```python
from build123d import *

# Parameters (mm, degrees)
SKETCH1_R                         = 30.48
BOSS_EXTRUDE1_DEPTH               = 25.4
F_1_4_28_TAPPED_HOLE1_D           = 5.4102
SKETCH7_R                         = 11.43
CUT_EXTRUDE2_DEPTH                = 12.7
F_1_4_CLEARANCE_HOLE1_D           = 6.5278
F_1_4_NPT_TAPPED_HOLE1_AT_2_COUNT = 2
F_1_4_NPT_TAPPED_HOLE1_AT_2_PITCH = 40.7035
CUT_EXTRUDE3_DEPTH                = 12.7
GASKET_SLOT_DEPTH                 = 1.016


with BuildPart() as part:
    # Sketch1 → Boss-Extrude1 (new body)
    with BuildSketch(Plane(origin=(0, 0, 0), x_dir=(1, 0, 0), z_dir=(0, 1, 0))):
        with Locations(Location((0, 0, 0), (0, 0, 270))):
            Circle(SKETCH1_R)
    extrude(amount=BOSS_EXTRUDE1_DEPTH)

    # 1/4-28 Tapped Hole1 (through all)
    with Locations(Plane(origin=(0, 25.4, 0), x_dir=(1, 0, 0), z_dir=(0, 1, 0))):
        with Locations((0, 0)):
            Hole(F_1_4_28_TAPPED_HOLE1_D / 2)

    # Sketch7 → Cut-Extrude2 (cut)
    with BuildSketch(Plane.XZ):
        with Locations(Location((0, 0, 0), (0, 0, 270))):
            Circle(SKETCH7_R)
    extrude(amount=-CUT_EXTRUDE2_DEPTH, mode=Mode.SUBTRACT)

    # 1/4 Clearance Hole1 (through all)
    with Locations(Plane(origin=(0, 25.4, 0), x_dir=(1, 0, 0), z_dir=(0, 1, 0))):
        with Locations((20.175514493, 15.615257641), (3.435452557, -25.280136906), (-3.435452557, 25.280136906), (-20.175514493, -15.615257641)):
            Hole(F_1_4_CLEARANCE_HOLE1_D / 2)

    # Sketch12 → 1/4 NPT Tapped Hole1 (revolve, cut)
    with BuildSketch(Plane(origin=(-18.83486521, 25.4, -7.709836613), x_dir=(0, 0, 1), z_dir=(1, 0, 0))):
        Polygon((0, 0), (0, 25.4), (5.5626, 25.4), (5.5626, 9.906), (6.557984794, 9.906), (6.8545837, 0), align=None)
    f_1_4_npt_tapped_hole1 = revolve(axis=Axis((-18.83486521, 31.75, -7.709836613), (0, -1, 0)), mode=Mode.SUBTRACT)

    # 1/4 NPT Tapped Hole1 at 2: 1/4 NPT Tapped Hole1 ×2
    with Locations(*[Vector(0.9254666163685309, 0, 0.37882917256645177) * (i * F_1_4_NPT_TAPPED_HOLE1_AT_2_PITCH) for i in range(1, F_1_4_NPT_TAPPED_HOLE1_AT_2_COUNT)]):
        add(f_1_4_npt_tapped_hole1, mode=Mode.SUBTRACT)

    # Sketch13 → Cut-Extrude3 (cut)
    with BuildSketch(Plane.XZ):
        with BuildLine():
            Line((-7.195822597, 8.880598919), (-22.336832207, -3.387945139))
            ThreePointArc((-22.336832207, -3.387945139), (-23.98286581, -9.817111768), (-18.30123054, -13.246780969))
            Line((-18.30123054, -13.246780969), (1.096509596, -11.377282923))
            ThreePointArc((1.096509596, -11.377282923), (4.330017442, -10.578083425), (7.195822597, -8.880598919))
            Line((7.195822597, -8.880598919), (22.336832207, 3.387945139))
            ThreePointArc((22.336832207, 3.387945139), (23.98286581, 9.817111768), (18.30123054, 13.246780969))
            Line((18.30123054, 13.246780969), (-1.096509596, 11.377282923))
            ThreePointArc((-1.096509596, 11.377282923), (-4.330017442, 10.578083425), (-7.195822597, 8.880598919))
        make_face()
    extrude(amount=-CUT_EXTRUDE3_DEPTH, mode=Mode.SUBTRACT)

    # Sketch16 → gasket slot (cut)
    with BuildSketch(Plane.XZ):
        with BuildLine():
            Line((18.008827981, 16.280723081), (-1.388912154, 14.411225036))
            ThreePointArc((-1.388912154, 14.411225036), (-5.48468876, 13.398905672), (-9.114708623, 11.24875863))
            Line((-9.114708623, 11.24875863), (-24.255718233, -1.019785427))
            ThreePointArc((-24.255718233, -1.019785427), (-26.803688057, -10.971783086), (-18.008827981, -16.280723081))
            Line((-18.008827981, -16.280723081), (1.388912154, -14.411225036))
            ThreePointArc((1.388912154, -14.411225036), (5.48468876, -13.398905672), (9.114708623, -11.24875863))
            Line((9.114708623, -11.24875863), (24.255718233, 1.019785427))
            ThreePointArc((24.255718233, 1.019785427), (26.803688057, 10.971783086), (18.008827981, 16.280723081))
        make_face()
        with BuildLine():
            Line((18.15502926, 14.763752025), (-1.242710875, 12.894253979))
            ThreePointArc((-1.242710875, 12.894253979), (-4.907353101, 11.988494548), (-8.15526561, 10.064678774))
            Line((-8.15526561, 10.064678774), (-23.29627522, -2.203865283))
            ThreePointArc((-23.29627522, -2.203865283), (-25.393276933, -10.394447427), (-18.15502926, -14.763752025))
            Line((-18.15502926, -14.763752025), (1.242710875, -12.894253979))
            ThreePointArc((1.242710875, -12.894253979), (4.907353101, -11.988494548), (8.15526561, -10.064678774))
            Line((8.15526561, -10.064678774), (23.29627522, 2.203865283))
            ThreePointArc((23.29627522, 2.203865283), (25.393276933, 10.394447427), (18.15502926, 14.763752025))
        make_face(mode=Mode.SUBTRACT)
    extrude(amount=-GASKET_SLOT_DEPTH, mode=Mode.SUBTRACT)


solid = part.part
```
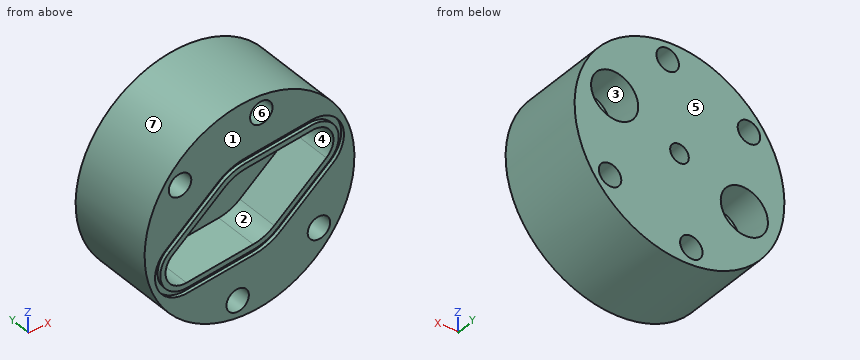
Can you work these out from the model? Positions are in its coordinate system, mm. Face numbers are marked on the shaded views. A direction names the side the tool comes from. Coordinates: 2 decimals unless noted, no trailing zeros. Write each loop counter-clockwise with the first axis right and the second up, starting at its lowest first coordinate (ties: lowest second). Pieces come first, ordered by that corner, then holes. Notation, with made-up numbers: M 35,-25.75 L 75,-25.75 A29 ccw 75,-3.75 Z; hole C -40,69 d8. An arc over 180 degrees is marked long. Answer as CSV lines item,"result".
Item 1: Imagine slicing it at B-B on z = 0. List the corners of the cut face in (x, y) for me.
Geometry results:
outline,"M -30.48,0 L -23,0 L -23,1.02 L -20.58,1.02 L -20.58,0 L -18.16,0 L -18.16,12.7 L -2.71,12.7 L -2.71,25.4 L -30.48,25.4 Z; M 2.71,12.7 L 18.16,12.7 L 18.16,0 L 20.58,0 L 20.58,1.02 L 23,1.02 L 23,0 L 30.48,0 L 30.48,25.4 L 2.71,25.4 Z"
Item 2: Imagine slicing it at D-D on x = 20. State how many separate pieces and enclosed holes the cut face has, plus the area to 3 significant figures.
Geometry results:
separate pieces,"3"
enclosed holes,"0"
area,"690 mm2"
Item 3: I'm going to push flat-ended pins straight in: P1, Ø4, axis at x = -21.5, z = -7.5, coming from the +Y side; P2, Ø13, axis at x = -3.5, z = 1, coming from the -Y side; P3, Ø18, axis at x = -18.83, z = -7.71, coming from the +Y side; P4, Ø4, axis at x = 20.5, z = 11, coming from the +Y side. Where does each tip first touch, or does it pass through?
Geometry results:
P1,"passes through"
P2,"stops at y = 12.7"
P3,"stops at y = 25.4"
P4,"stops at y = 15.49"
Item 4: Imagine slicing it at A-A on y = 21.5. List the corners of the cut face in (x, z) for me, plus the area to 3 significant figures.
Geometry results:
outline,"C 0,0 d60.96; hole C -18.83,-7.71 d13.48; hole C -20.18,15.62 d6.53; hole C -3.44,-25.28 d6.53; hole C 0,0 d5.41; hole C 3.44,25.28 d6.53; hole C 18.83,7.71 d13.48; hole C 20.18,-15.62 d6.53"
area,"2,480 mm2"
Item 5: Imagine slicing it at C-C on y = 11.75. List the corners of the cut face in (x, z) for me, plus the area to 3 significant figures.
Geometry results:
outline,"C 0,0 d60.96; hole C -20.18,15.62 d6.53; hole M -22.34,-3.39 A5.56 ccw -18.3,-13.25 L 1.1,-11.38 A11.43 ccw 7.2,-8.88 L 22.34,3.39 A5.56 ccw 18.3,13.25 L -1.1,11.38 A11.43 ccw -7.2,8.88 Z; hole C -3.44,-25.28 d6.53; hole C 3.44,25.28 d6.53; hole C 20.18,-15.62 d6.53"
area,"1,970 mm2"
Item 6: We'd pull the mould along X, two halves only. Please class the marked faces 4, 5, 6 and 7: +X half, -X half, draft (parallel to the pull), parting line (faces both ways), or undercut.
Geometry results:
face 4,"undercut"
face 5,"draft"
face 6,"undercut"
face 7,"parting line"
Item 7: On a 3-axis mill with a long thin cutter (end or side, diameter ignored), from which of +Z, -Z, +X, -X, +Y, -Y can I reach the whole of each face in a straight line? I mean the marked faces 1, 2 and 3. Say none if no direction works.
Geometry results:
face 1,"+Z, -Z, +X, -X, -Y"
face 2,"-Y"
face 3,"+Y"
Item 8: Please list where these lines run through material, in increasing order: line 1 along X through (y, z) = (24, -2); line 2 along Z through (x, y) = (19.5, 14.75); line 3 along Z through (x, y) = (22.5, 6.25).
Geometry results:
line 1,"x = -30.41 to -22.55, -15.12 to -1.82, 1.82 to 30.41"
line 2,"z = -23.43 to -18.81, -12.42 to 2.19, 13.23 to 23.43"
line 3,"z = -20.56 to -17.91, -13.32 to 3.53, 11.89 to 20.56"
